```python
from build123d import *

# Parameters (mm, degrees)
SKETCH2_W           = 110
SKETCH2_H           = 82
BOSS_EXTRUDE1_DEPTH = 5
SKETCH13_W          = 20.02707563
SKETCH13_H          = 50.8
CUT_EXTRUDE12_DEPTH = 5
SKETCH14_W          = 2.498354032
SKETCH14_H          = 82
CUT_EXTRUDE13_DEPTH = 2.5
SKETCH15_W          = 107.501645968
SKETCH15_H          = 2.500122833
CUT_EXTRUDE14_DEPTH = 2.5
SKETCH16_W          = 107.501645968
SKETCH16_H          = 2.501703456
CUT_EXTRUDE15_DEPTH = 2.5
SKETCH18_W          = 2.5
SKETCH18_H          = 76.998173711
CUT_EXTRUDE18_DEPTH = 2.5
SKETCH19_W          = 7.5
SKETCH19_H          = 9.5
CUT_EXTRUDE19_DEPTH = 10
SKETCH20_W          = 7.5
SKETCH20_H          = 9.5
CUT_EXTRUDE20_DEPTH = 10
CUT_EXTRUDE21_DEPTH = 8
SKETCH22_W          = 7
SKETCH22_H          = 13
CUT_EXTRUDE22_DEPTH = 10


with BuildPart() as part:
    # Sketch2 → Boss-Extrude1 (new body)
    with BuildSketch(Plane.XY):
        Rectangle(SKETCH2_W, SKETCH2_H)
    extrude(amount=BOSS_EXTRUDE1_DEPTH)

    # Sketch13 → Cut-Extrude12 (cut)
    with BuildSketch(Plane.XY.offset(5)):
        with Locations((-36.986462185, -0.9)):
            Rectangle(SKETCH13_W, SKETCH13_H)
    extrude(amount=-CUT_EXTRUDE12_DEPTH, mode=Mode.SUBTRACT)

    # Sketch14 → Cut-Extrude13 (cut)
    with BuildSketch(Plane.XY.offset(5)):
        with Locations((-53.750822984, 0)):
            Rectangle(SKETCH14_W, SKETCH14_H)
    extrude(amount=-CUT_EXTRUDE13_DEPTH, mode=Mode.SUBTRACT)

    # Sketch15 → Cut-Extrude14 (cut)
    with BuildSketch(Plane.XY.offset(5)):
        with Locations((1.249177016, -39.749938583)):
            Rectangle(SKETCH15_W, SKETCH15_H)
    extrude(amount=-CUT_EXTRUDE14_DEPTH, mode=Mode.SUBTRACT)

    # Sketch16 → Cut-Extrude15 (cut)
    with BuildSketch(Plane.XY.offset(5)):
        with Locations((1.249177016, 39.749148272)):
            Rectangle(SKETCH16_W, SKETCH16_H)
    extrude(amount=-CUT_EXTRUDE15_DEPTH, mode=Mode.SUBTRACT)

    # Sketch18 → Cut-Extrude18 (cut)
    with BuildSketch(Plane.XY.offset(5)):
        with Locations((53.75, -0.000790311)):
            Rectangle(SKETCH18_W, SKETCH18_H)
    extrude(amount=-CUT_EXTRUDE18_DEPTH, mode=Mode.SUBTRACT)

    # Sketch19 → Cut-Extrude19 (cut)
    with BuildSketch(Plane.XY.offset(5)):
        Polygon((6.1, -34.499877167), (13.6, -34.499877167), (13.6, -24.999877167), (21.1, -24.999877167), (21.1, -15.499877167), (6.1, -15.499877167), align=None)
        with Locations((17.35, -29.749877167)):
            Rectangle(SKETCH19_W, SKETCH19_H)
    extrude(amount=-CUT_EXTRUDE19_DEPTH, mode=Mode.SUBTRACT)

    # Sketch20 → Cut-Extrude20 (cut)
    with BuildSketch(Plane.XY.offset(5)):
        Polygon((31.4, -24.999877167), (38.9, -24.999877167), (38.9, -15.499877167), (23.9, -15.499877167), (23.9, -34.499877167), (31.4, -34.499877167), align=None)
        with Locations((35.15, -29.749877167)):
            Rectangle(SKETCH20_W, SKETCH20_H)
    extrude(amount=-CUT_EXTRUDE20_DEPTH, mode=Mode.SUBTRACT)

    # Sketch21 → Cut-Extrude21 (cut)
    with BuildSketch(Plane.XY.offset(5)):
        with BuildLine():
            ThreePointArc((1.498354032, -24.499877167), (-6.501645968, -16.499877167), (-14.501645968, -24.499877167))
            Line((-14.501645968, -24.499877167), (-6.501645968, -24.499877167))
            Line((-6.501645968, -24.499877167), (-6.501645968, -32.499877167))
            ThreePointArc((-6.501645968, -32.499877167), (-0.844791718, -30.156731417), (1.498354032, -24.499877167))
        make_face()
        with BuildLine():
            Line((-6.501645968, -24.499877167), (-14.501645968, -24.499877167))
            ThreePointArc((-14.501645968, -24.499877167), (-12.158500217, -30.156731417), (-6.501645968, -32.499877167))
            Line((-6.501645968, -32.499877167), (-6.501645968, -24.499877167))
        make_face()
    extrude(amount=-CUT_EXTRUDE21_DEPTH, mode=Mode.SUBTRACT)

    # Sketch22 → Cut-Extrude22 (cut)
    with BuildSketch(Plane.XY.offset(5)):
        with Locations((32.75, 24.298296544)):
            Rectangle(SKETCH22_W, SKETCH22_H)
    extrude(amount=-CUT_EXTRUDE22_DEPTH, mode=Mode.SUBTRACT)


solid = part.part
```
Here's how the part is built. I have some questions about the finished solid (model axes, mm). A direction names the side the tool comes from. Give positions to 0.01 mm unless a question says otherwise; leave off trailing zeros. Write each loop counter-clockwise with the first axis right and the second up, starting at its lowest first coordinate (ties: lowest second). Pieces come first, ordered by that corner, then holes. Notation, with made-up numbers: M 37,30 L 90,30 A23 ccw 90,59 Z; hole C 36,33 d5. An arc over 180 degrees is marked long. Put each result on its own line as item: value. Start each with the question number.
Item 1: On a 3-axis mill with a long thin cutter (end or side, diameter ignored), from which of +Z, -Z, +X, -X, +Y, -Y can I reach the whole of each face in a straight line? I mean faces 1 (the flat face through (-1, 38.498, 4)), 2 (the flat face through (-37, -26.3, 3)), 3 (the flat face through (-1, 41, 1)). Say none if no direction works.
Item 2: If we section it at D-D, the plane y = -19: Write out the boundary of the cut face in (x, z).
Item 3: Will these pins go through, and if not, where does the flat tip stop? pin 1 (2 mm diameter, centred on x = 38.5, y = -27.5, fed in from -Z); pin 2 (1.2 mm diameter, centred on y = -3.5, z = 4.5, fed in from -X); pin 3 (1.2 mm diameter, centred on y = -5, z = 3.5, fed in from +X).
Item 4: If we section it at B-B, the plane y = 4: Write out the boundary of the cut face in (x, z).
Item 5: Thinking about a two-plate mould opening in Y: for faces 4 (the flat face through (29.25, 24, 3)), 5 (the flat face through (-1, -41, 1)), 6 (the flat face through (-4, -39, 2.5)), which applies, +Y half, -Y half, draft (parallel to the pull), parting line (faces both ways), or undercut?
Item 6: If we section it at C-C, the plane z = 3.6: Write out the boundary of the cut face in (x, y), then the cut area to 3 significant figures.
Item 7: I need wall thicknesses on L1, parallel to Y at x = -35.5, z = 3.3; L2, parallel to Y at x = 16.5, z = 1; L3, parallel to X at y = -24, z = 3.55. Which ranges of each line are inside material? Lowest first, please. Write a range as from..to.
Item 8: If we section it at A-A, the plane x = 37.5: Write out the boundary of the cut face in (y, z), then the cut area to 3 significant figures.
Values:
1. face 1: +Z, +X, -X, +Y
1. face 2: +Z, -Z
1. face 3: +Z, -Z, +X, -X, +Y
2. outline: M -55,0 L -47,0 L -47,5 L -52.5,5 L -52.5,2.5 L -55,2.5 Z; M -26.97,0 L -12.31,0 L -12.31,5 L -26.97,5 Z; M -0.69,0 L 6.1,0 L 6.1,5 L -0.69,5 Z; M 21.1,0 L 23.9,0 L 23.9,5 L 21.1,5 Z; M 38.9,0 L 55,0 L 55,2.5 L 52.5,2.5 L 52.5,5 L 38.9,5 Z
3. pin 1: z = 0
3. pin 2: x = -52.5
3. pin 3: x = 52.5
4. outline: M -55,0 L -47,0 L -47,5 L -52.5,5 L -52.5,2.5 L -55,2.5 Z; M -26.97,0 L 55,0 L 55,2.5 L 52.5,2.5 L 52.5,5 L -26.97,5 Z
5. face 4: undercut
5. face 5: -Y half
5. face 6: draft
6. outline: M -52.5,-38.5 L 52.5,-38.5 L 52.5,38.5 L -52.5,38.5 Z; hole M -47,-26.3 L -26.97,-26.3 L -26.97,24.5 L -47,24.5 Z; hole C -6.5,-24.5 d16; hole M 6.1,-34.5 L 21.1,-34.5 L 21.1,-15.5 L 6.1,-15.5 Z; hole M 23.9,-34.5 L 38.9,-34.5 L 38.9,-15.5 L 23.9,-15.5 Z; hole M 29.25,17.8 L 36.25,17.8 L 36.25,30.8 L 29.25,30.8 Z
6. area: 6,210 mm²
7. L1: -38.5..-26.3, 24.5..38.5
7. L2: -41..-34.5, -15.5..41
7. L3: -52.5..-47, -26.97..-14.49, 1.48..6.1, 21.1..23.9, 38.9..52.5
8. outline: M -41,0 L -34.5,0 L -34.5,5 L -38.5,5 L -38.5,2.5 L -41,2.5 Z; M -15.5,0 L 41,0 L 41,2.5 L 38.5,2.5 L 38.5,5 L -15.5,5 Z
8. area: 302 mm²
